from build123d import *

# Parameters (mm, degrees)
F0_R     = 15.875
F1_DEPTH = 50.8


with BuildPart() as f1:
    # F0 (on Front) → F1 (new body)
    with BuildSketch(Plane.XZ):
        with BuildLine():
            ThreePointArc((10.780709, -43.122834), (35.035732, -27.355073), (44.45, 0))
            ThreePointArc((44.45, 0), (35.035732, 27.355073), (10.780709, 43.122834))
            ThreePointArc((10.780709, 43.122834), (-44.45, 0), (10.780709, -43.122834))
        make_face()
        with BuildLine():
            ThreePointArc((-24.593444, 6.35), (0, 25.4), (24.593444, 6.35))
            Line((24.593444, 6.35), (31.75, 6.35))
            Line((31.75, 6.35), (31.75, -6.35))
            Line((31.75, -6.35), (24.593444, -6.35))
            ThreePointArc((24.593444, -6.35), (0, -25.4), (-24.593444, -6.35))
            Line((-24.593444, -6.35), (-31.75, -6.35))
            Line((-31.75, -6.35), (-31.75, 6.35))
            Line((-31.75, 6.35), (-24.593444, 6.35))
        make_face(mode=Mode.SUBTRACT)
        with BuildLine():
            ThreePointArc((10.780709, 43.122834), (35.035732, 27.355073), (44.45, 0))
            ThreePointArc((44.45, 0), (35.035732, -27.355073), (10.780709, -43.122834))
            Line((10.780709, -43.122834), (84.705567, -24.64162))
            ThreePointArc((84.705567, -24.64162), (53.145162, 0), (84.705567, 24.64162))
            Line((84.705567, 24.64162), (10.780709, 43.122834))
        make_face()
        with BuildLine():
            ThreePointArc((103.945162, 0), (98.56558, 15.63147), (84.705567, 24.64162))
            ThreePointArc((84.705567, 24.64162), (53.145162, 0), (84.705567, -24.64162))
            ThreePointArc((84.705567, -24.64162), (98.56558, -15.63147), (103.945162, 0))
        make_face()
        with Locations((78.545162, 0)):
            Circle(F0_R, mode=Mode.SUBTRACT)
        with BuildLine():
            ThreePointArc((-24.593444, -6.35), (-25.4, 0), (-24.593444, 6.35))
            Line((-24.593444, 6.35), (-31.75, 6.35))
            Line((-31.75, 6.35), (-31.75, -6.35))
            Line((-31.75, -6.35), (-24.593444, -6.35))
        make_face()
    extrude(amount=F1_DEPTH)


solid = f1.part
Read the model definition and answer for the solid it produces. Units are mm, in the model's axes. A direction names the side the tool comes from. Give positions to 0.01 mm unless a question says otherwise; leave off trailing zeros. Write each loop counter-clockwise with the first axis right and the second up, starting at its lowest first coordinate (ties: lowest second). Pieces come first, ordered by that corner, then holes. Notation, with made-up numbers: (73, 86) - (92, 86) arc R20 cw to (92, 91) - close; hole circle Ø6 at (83, 21.25). An arc over 180 degrees is marked (long way). Answer in a Markdown table with one row per item. Add a question column.
Item 1: A tool of negligible diameter and unlimited length cuts with its end or side. For faces 4 (the face through (28, -25, -6.35)), 5 (the face through (47.23, -25.04, -34.01)), from which of +Z, -Z, +X, -X, +Y, -Y can it reach the whole face along a straight path? Write none if from no direction.
Item 2: Section C-C, the plane z = -18 is taken. Write down the section's boundary in (x, y).
Item 3: Determine the mould class of faces 1 (the face through (48.261, -25.044, 33.753)), 2 (the face through (29, -50.8, -9)), 3 (the face through (28, -25, 6.35)) for opening direction X: pulls with the +X half, pulls with the -X half, needs draft (parallel to the pull), parting line crosses it, or undercut.
Item 4: Section B-B, the plane x = 0 is taken. Write down the section's boundary in (y, z).
Item 5: Section A-A, the plane y = -38 is taken. Write down the section's boundary in (x, z) (3 decimals).
Item 6: Section D-D, the plane z = 11 is taken. Write down the section's boundary in (x, y).
Item 7: Find the intervals of material crossed by L1, parallel to Z at x = -1, y = -12.5; L2, parallel to X at y = -34, z = 2.5; L3, parallel to Z at x = -2, y = -5, in increasing order.
Item 8: Flat-ended cylindrical pins translate along their axes: P1, Ø1.5, axis at x = 16.5, y = -31.5, coming from the -Z side; P2, Ø12, axis at y = -13, z = -23.5, coming from the -X side; P3, Ø10, axis at x = -25, y = -28, coming from the -Z side. Find the tip coordinate at first contact, or state that the pin passes through.
Recorded:
| question | item | result |
|---|---|---|
| 1 | face 4 | +Y, -Y |
| 1 | face 5 | -Z, +X, +Y, -Y |
| 2 | outline | (-40.64, -50.8) - (-17.92, -50.8) - (-17.92, 0) - (-40.64, 0) - close; (17.92, -50.8) - (96.47, -50.8) - (96.47, 0) - (17.92, 0) - close |
| 3 | face 1 | pulls with the +X half |
| 3 | face 2 | needs draft |
| 3 | face 3 | undercut |
| 4 | outline | (-50.8, -44.45) - (0, -44.45) - (0, -25.4) - (-50.8, -25.4) - close; (-50.8, 25.4) - (0, 25.4) - (0, 44.45) - (-50.8, 44.45) - close |
| 5 | outline | (10.781, -43.123) - (84.706, -24.642) arc R25.4 ccw to (103.945, 0) arc R25.4 ccw to (84.706, 24.642) - (10.781, 43.123) arc R44.45 ccw (long way) to start; hole (-24.593, -6.35) arc R25.4 ccw to (24.593, -6.35) - (31.75, -6.35) - (31.75, 6.35) - (24.593, 6.35) arc R25.4 ccw to (-24.593, 6.35) arc R25.4 ccw to start; hole circle Ø31.75 at (78.545, 0) |
| 6 | outline | (-43.07, -50.8) - (-22.89, -50.8) - (-22.89, 0) - (-43.07, 0) - close; (22.89, -50.8) - (67.1, -50.8) - (67.1, 0) - (22.89, 0) - close; (89.99, -50.8) - (101.44, -50.8) - (101.44, 0) - (89.99, 0) - close |
| 7 | L1 | z = -44.44 to -25.38, 25.38 to 44.44 |
| 7 | L2 | x = -44.38 to -25.28, 31.75 to 62.87, 94.22 to 103.82 |
| 7 | L3 | z = -44.4 to -25.32, 25.32 to 44.4 |
| 8 | P1 | stops at z = -41.88 |
| 8 | P2 | stops at x = -40.86 |
| 8 | P3 | stops at z = -39.7 |
